Autodesk Inventor part; units mm, degrees
ref_plane "YZ Plane" through (0, 0, 0) normal (1, 0, 0) x (0, 1, 0)
ref_plane "XZ Plane" through (0, 0, 0) normal (0, 1, 0) x (-1, 0, 0)
ref_plane "XY Plane" through (0, 0, 0) normal (0, 0, 1) x (1, 0, 0)
sketch "Sketch1" plane through (0, 0, 0) normal (0, 1, 0) x (-1, 0, 0)
  line L0 (115.6192, -60.316) -> (18.6192, -60.316)
  line L1 (18.6192, -60.316) -> (18.6192, -90.316)
  line L2 (18.6192, -90.316) -> (115.6192, -90.316)
  line L3 (115.6192, -90.316) -> (115.6192, -60.316)
  line L4 (115.6192, -60.316) -> (18.6192, -90.316) construction
  line L5 (18.6192, -60.316) -> (115.6192, -90.316) construction
  line L6 (113.2192, -60.316) -> (113.2192, -90.316)
  line L7 (111.2192, -60.316) -> (111.2192, -90.316)
  line L8 (25.6192, -60.316) -> (25.6192, -90.316)
  line L9 (23.6192, -60.316) -> (23.6192, -90.316)
  line L10 (65.6192, -90.316) -> (65.6192, -60.316)
  line L11 (68.1192, -90.316) -> (68.1192, -60.316)
  line L12 (20.6192, -90.316) -> (20.6192, -60.316)
  point P0 (0, 0)
  point P1 (67.1192, -75.316)
  dimension "d0" = 97
  dimension "d1" = 30
  dimension "d2" = 2.4
  dimension "d3" = 2
  dimension "d4" = 5
  dimension "d5" = 2
  dimension "d24" = 47
  dimension "d25" = 2.5
  dimension "d28" = 2
  dimension "d29" = 3
extrude "Extrusion1" add sketch "Sketch1" along normal blind 3 contours L7 L2 L11 L0 | L10 L2 L8 L0 | L9 L2 L12 L0
extrude "Extrusion2" add sketch "Sketch1" along normal blind 16 contours L6 L2 L7 L0
extrude "Extrusion8" add sketch "Sketch1" along normal blind 16 contours L11 L2 L10 L0
extrude "Extrusion4" add sketch "Sketch1" along normal blind 16 contours L8 L2 L9 L0
extrude "Extrusion5" add sketch "Sketch1" along normal blind 3 contours L9 L2 L12 L0 | L12 L2 L1 L0
extrude "Extrusion9" add sketch "Sketch1" along normal blind 16 contours L12 L2 L1 L0
sketch "Sketch2" plane through (-18.6192, 16, -60.316) normal (1, 0, 0) x (0, 0, -1)
  line L0 (30, -13) -> (0, -13) construction
  line L1 (30, -13) -> (30, 0) construction
  line L2 (0, 0) -> (30, 0) construction
  line L3 (0, -13) -> (0, 0) construction
  line L4 (0, 0) -> (30, 0) construction
  line L5 (15, 0) -> (15, -13) construction
  line L6 (30, -13) -> (0, -13) construction
  circle A0 centre (15, 0) radius 4.5
  point P0 (-60.316, -16)
  dimension "d18" = 9
extrude "Extrusion6" cut sketch "Sketch2" against normal up to surface (49.5 mm away)
sketch "Sketch3" plane through (-113.2192, 16, -90.316) normal (-1, 0, 0) x (0, 0, 1)
  line L0 (30, 0) -> (0, 0)
  circle A0 centre (15, 0) radius 3.5
  point P0 (90.316, -16)
  dimension "d19" = 7
extrude "Extrusion7" cut sketch "Sketch3" against normal up to surface (2 mm away)
properties part number "Hamilton 10 micL syringe holder_3DPrint"
For this review, take the finished solid that the model builds, in its own axes (mm). A direction names the side the tool comes from. Give positions to 0.01 mm unless a question says otherwise; leave off trailing zeros. Order: outer loops, then holes, each group sorted by start corner. A loop starts at its lowest first (then second) coordinate and runs counter-clockwise, first axis right, second up. Notation, with made-up numbers: M 81.5,61 L 119.5,61 A27 ccw 119.5,98 Z; hole C 35.5,-3.5 d5. An arc over 180 degrees is marked long. Answer in a Markdown table with one row per item. Add a question column.
(1) Consider section A-A on y = 7.5. State the section outline as (x, z) points, and give its area (3 significant figures).
(2) Consider section B-B on z = -65. State the section outline as (x, y) points.
(3) For pin 1 (3 mm diameter, centred on x = -45.5, y = 5, fed in from +Z); pin 2 (6 mm diameter, centred on x = -38, z = -66, fed in from +Y), all flat-tipped, find the tip position at first contact; note any pin that passes through.
(4) For faces 4 (the face through (-66.9, 11.5, -75.2)), 5 (the face through (-67, 16, -85)), 6 (the face through (-23.619, 9, -75)), list the 3-axis set-ups (+Z, -Z, +X, -X, +Y, -Y) from which the entire face can be reached by the end or side of a thin tool; tool diameter is ignored.
(5) Consider section C-C on x = -67. State the section outline as (y, z) points, and give its area (3 significant figures).
(6) Mouldability with a two-part tool opening along Z and no side actions: class faces 1 (the face through (-20, 16, -65)), 2 (the face through (-112.2, 12.5, -75.4)), 3 (the face through (-62.2, 2.6, -90.316)) as +Z half, -Z half, draft (parallel to the pull), parting line (faces both ways), or undercut.
(7) Wall thickness on probe 1 along X at (y, z) = (10, -81.5); probe 2 along Y at (x, z) = (-55, -75.5); probe 3 along Z at (x, y) = (-66.5, 13): over which ranges is each line inside the solid? List them lowest first. Write a range as [from, to].
Evaluation:
| question | item | result |
|---|---|---|
| 1 | outline | M -113.22,-90.32 L -111.22,-90.32 L -111.22,-60.32 L -113.22,-60.32 Z; M -68.12,-90.32 L -65.62,-90.32 L -65.62,-60.32 L -68.12,-60.32 Z; M -25.62,-90.32 L -23.62,-90.32 L -23.62,-60.32 L -25.62,-60.32 Z; M -20.62,-90.32 L -18.62,-90.32 L -18.62,-60.32 L -20.62,-60.32 Z |
| 1 | area | 255 mm^2 |
| 2 | outline | M -113.22,0 L -18.62,0 L -18.62,16 L -20.62,16 L -20.62,3 L -23.62,3 L -23.62,16 L -25.62,16 L -25.62,3 L -65.62,3 L -65.62,16 L -68.12,16 L -68.12,3 L -111.22,3 L -111.22,16 L -113.22,16 Z |
| 3 | pin 1 | passes through |
| 3 | pin 2 | stops at y = 3 |
| 4 | face 4 | +X, +Y |
| 4 | face 5 | +Z, -Z, +X, -X, +Y |
| 4 | face 6 | +Z, -Z, +Y |
| 5 | outline | M 0,-90.32 L 16,-90.32 L 16,-79.82 A4.5 cw 16,-70.82 L 16,-60.32 L 0,-60.32 Z |
| 5 | area | 448 mm^2 |
| 6 | face 1 | draft |
| 6 | face 2 | undercut |
| 6 | face 3 | -Z half |
| 7 | probe 1 | x = [-113.22, -111.22], [-68.12, -65.62], [-25.62, -23.62], [-20.62, -18.62] |
| 7 | probe 2 | y = [0, 3] |
| 7 | probe 3 | z = [-90.32, -78.67], [-71.96, -60.32] |
